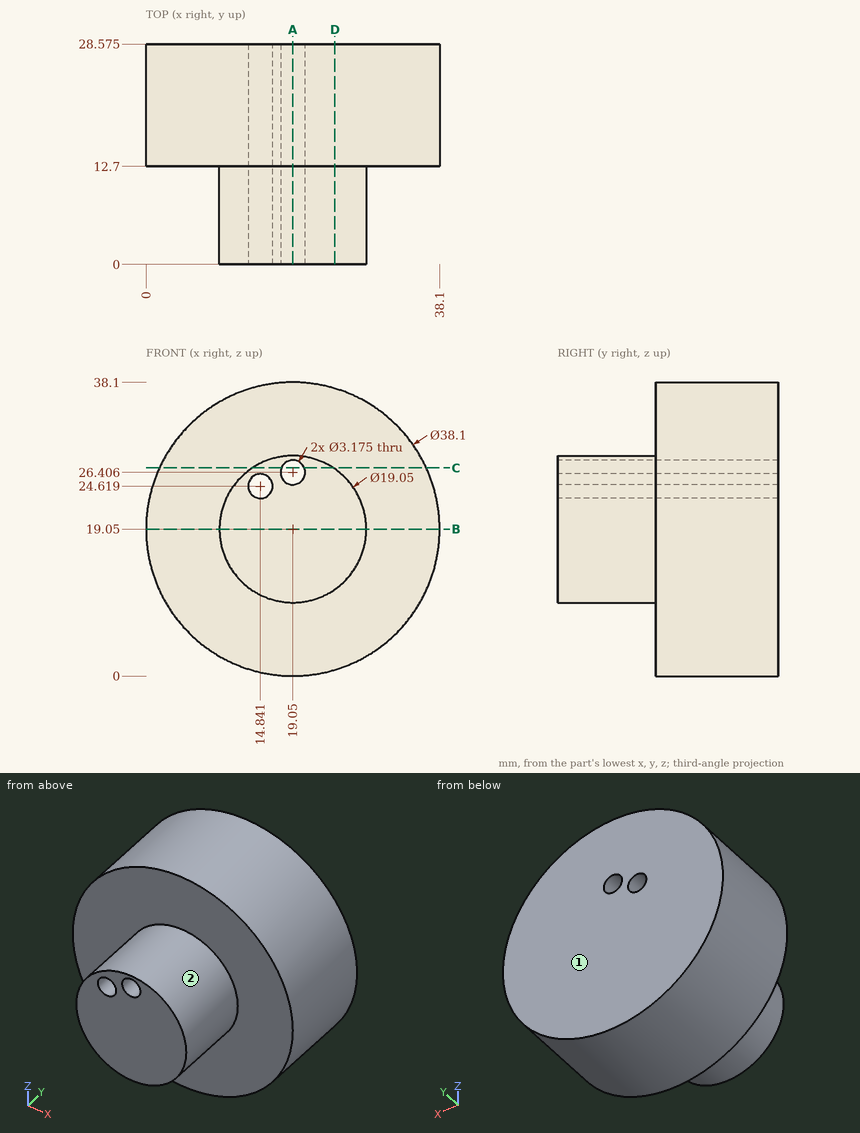
Could you check a few things on this drawing? It's one solid part, dimensions in mm from its lowest x, y, z. A direction names the side the tool comes from. Round coordinates to 2 decimals unless told otherwise and drop trailing zeros. Write each loop counter-clockwise with the first axis right and the second up, starting at its lowest first coordinate (ties: lowest second). Pieces come first, ordered by that corner, then holes. Notation, with made-up numbers: M -27.75,15 L -2.75,15 A28 cw -2.75,51 Z; hole C 26.25,70 d8. An arc over 180 degrees is marked long. Answer as CSV lines item,"result". Start each with the question number.
1. I'm going to push flat-ended pins straight in: pin 1 Ø6 at (x, y) = (15, 12.5) entering from -Z; pin 2 Ø11.5 at (x, z) = (24.5, 17.5) entering from -Y; pin 3 Ø1.5 at (x, y) = (24, 4.5) entering from +Z; pin 4 Ø5 at (y, z) = (14, 27) entering from +X. Where does each tip first touch, or does it pass through?
2. Suppose I cut it at A-A on x = 19.05. Write out the boundary of the cut face in (y, z) (1 decimal).
3. I need wall thicknesses on probe 1 along Z at (x, y) = (19.05, 15.5); probe 2 along Y at (x, z) = (28, 28.5) (1 decimal); probe 3 along X at (y, z) = (7, 19.5). Which ranges of each line are inside material? Lowest first, please.
4. Suppose I cut it at D-D on x = 24.5. Write out the boundary of the cut face in (y, z) (1 decimal), then the cut area to 3 significant figures.
5. Suppose I cut it at C-C on z = 27. Write out the boundary of the cut face in (x, y) (1 decimal), then the cut area to 3 significant figures.
6. On a 3-axis mill with a long thin cutter (end or side, diameter ignored), from which of +Z, -Z, +X, -X, +Y, -Y can I reach the whole of each face in a straight line? I mean the marked faces 1 and 2. Say none if no direction works.
7. Suppose I cut it at B-B on z = 19.05. Write out the boundary of the cut face in (x, y) (1 decimal).
Check result:
1,pin 1,"stops at z = 0.03"
1,pin 2,"stops at y = 0"
1,pin 3,"stops at z = 27.6"
1,pin 4,"stops at x = 37.3"
2,outline,"M 0,9.5 L 12.7,9.5 L 12.7,0 L 28.6,0 L 28.6,24.8 L 0,24.8 Z; M 0,28 L 28.6,28 L 28.6,38.1 L 12.7,38.1 L 12.7,28.6 L 0,28.6 Z"
3,probe 1,"z = 0 to 24.82, 27.99 to 38.1"
3,probe 2,"y = 12.7 to 28.6"
3,probe 3,"x = 9.54 to 28.56"
4,outline,"M 0,11.2 L 12.7,11.2 L 12.7,0.8 L 28.6,0.8 L 28.6,37.3 L 12.7,37.3 L 12.7,26.9 L 0,26.9 Z"
4,area,"778 mm2"
5,outline,"M 1.7,12.7 L 13.8,12.7 L 13.8,0 L 17.6,0 L 17.6,28.6 L 1.7,28.6 Z; M 20.5,0 L 24.3,0 L 24.3,12.7 L 36.4,12.7 L 36.4,28.6 L 20.5,28.6 Z"
5,area,"599 mm2"
6,face 1,"+Z, -Z, +X, -X, +Y"
6,face 2,"-Y"
7,outline,"M 0,12.7 L 9.5,12.7 L 9.5,0 L 28.6,0 L 28.6,12.7 L 38.1,12.7 L 38.1,28.6 L 0,28.6 Z"
